Check sheet for the modelled part. Datum: model origin and axes. Units: mm. Give positions to 0.01 mm unless a question says otherwise; leave off trailing zeros. Order: outer loops, then holes, each group sorted by start corner. A loop starts at its lowest first (then second) coordinate and runs counter-clockwise, first axis right, second up. Notation, with made-up numbers: M 55,65.25 L 75,65.25 A18 ccw 75,98.25 Z; hole C 49.25,81 d10. An arc over 180 degrees is marked long. Answer in a Markdown table with one row per item. Add a question column.
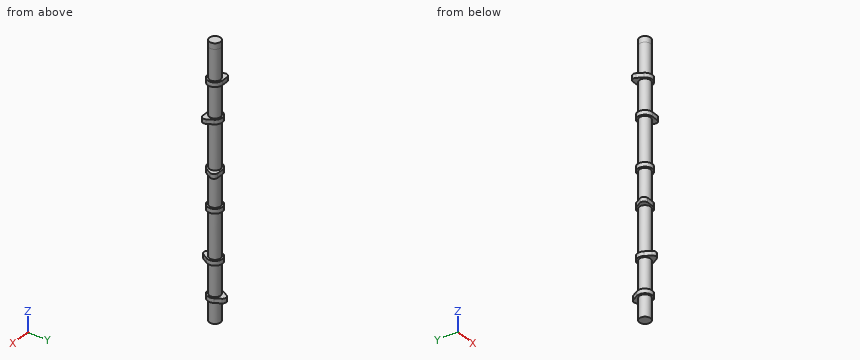
from build123d import *

# Parameters (mm, degrees)
BOSS_EXTRUDE1_DEPTH   = 3.81
BODY_MOVE_COPY2_ANGLE = 180
SKETCH2_R             = 9.5
BOSS_EXTRUDE2_DEPTH   = 146.05
LPATTERN1_COUNT       = 3
LPATTERN1_PITCH       = 146.05
BODY_MOVE_COPY3_ANGLE = 120
BODY_MOVE_COPY4_ANGLE = 120
BOSS_EXTRUDE3_START   = 27.94
SKETCH3_R             = 9.5
BOSS_EXTRUDE3_DEPTH   = 27.94
SKETCH4_R             = 9.5
CUT_EXTRUDE1_DEPTH    = 16.94
SKETCH5_R             = 9.5
BOSS_EXTRUDE4_DEPTH   = 10


with BuildPart() as part:
    # Sketch1 → Boss-Extrude1 (new, symmetric)
    with BuildSketch(Plane.XY):
        with BuildLine():
            Line((-5.499261314, 15.875), (-10.998522628, 6.35))
            ThreePointArc((-10.998522628, 6.35), (0, -12.7), (10.998522628, 6.35))
            Line((10.998522628, 6.35), (5.499261314, 15.875))
            ThreePointArc((5.499261314, 15.875), (0, 19.05), (-5.499261314, 15.875))
        make_face()
    extrude(amount=BOSS_EXTRUDE1_DEPTH, both=True)


with BuildPart() as body_2:
    # Body-Move_Copy1: copy of part
    add(part.part.moved(Location((0, 0, 60.96))))


with BuildPart() as body_2_1:
    # Body-Move_Copy2: moved
    add(body_2.part.rotate(Axis((0, 0, 0), (0, 0, 1)), BODY_MOVE_COPY2_ANGLE))


with BuildPart() as part_1:
    add(part.part)

    add(body_2_1.part)  # Boss-Extrude2 merges body 2
    # Sketch2 → Boss-Extrude2 (add)
    with BuildSketch(Plane(origin=(0, 0, -29.21), x_dir=(-1, 0, 0), z_dir=(0, 0, -1))):
        with Locations(Location((0, 0, 0), (0, 0, 180))):
            Circle(SKETCH2_R)
    extrude(amount=-BOSS_EXTRUDE2_DEPTH)


with BuildPart() as lpattern1_1:
    # LPattern1: pattern copy
    add(part_1.part.moved(Location(Vector(0, 0, 1) * (1 * LPATTERN1_PITCH))))


with BuildPart() as lpattern1_2:
    # LPattern1: pattern copy
    add(part_1.part.moved(Location(Vector(0, 0, 1) * (2 * LPATTERN1_PITCH))))


with BuildPart() as lpattern1_1_1:
    # Body-Move_Copy3: moved
    add(lpattern1_1.part.rotate(Axis((0, 0, 0), (0, 0, 1)), BODY_MOVE_COPY3_ANGLE))


with BuildPart() as lpattern1_2_1:
    # Body-Move_Copy4: moved
    add(lpattern1_2.part.rotate(Axis((0, 0, 0), (0, 0, -1)), BODY_MOVE_COPY4_ANGLE))


with BuildPart() as part_2:
    add(part_1.part)

    # Sketch3 → Boss-Extrude3 (add)
    with BuildSketch(Plane(origin=(0, 0, -29.21), x_dir=(-1, 0, 0), z_dir=(0, 0, -1)).offset(BOSS_EXTRUDE3_START)):
        with Locations(Location((0, 0, 0), (0, 0, 180))):
            Circle(SKETCH3_R)
    extrude(amount=-BOSS_EXTRUDE3_DEPTH)


with BuildPart() as lpattern1_2_2:
    add(lpattern1_2_1.part)

    # Combine1: union LPattern1_1, part
    add(lpattern1_1_1.part)
    add(part_2.part)

    # Sketch4 → Cut-Extrude1 (cut)
    with BuildSketch(Plane(origin=(0, 0, -57.15), x_dir=(-1, 0, 0), z_dir=(0, 0, -1))):
        Circle(SKETCH4_R)
    extrude(amount=-CUT_EXTRUDE1_DEPTH, mode=Mode.SUBTRACT)

    # Sketch5 → Boss-Extrude4 (add)
    with BuildSketch(Plane.XY.offset(408.94)):
        with Locations(Location((0, 0, 0), (0, 0, 180))):
            Circle(SKETCH5_R)
    extrude(amount=BOSS_EXTRUDE4_DEPTH)


solid = lpattern1_2_2.part
Q1. Thickness scan on probe 1 along Z at (x, y) = (3.5, 10); probe 2 along Z at (x, y) = (-11, -6.5); probe 3 along X at (y, z) = (0, 239). Record the ranges inside material, lowest first.
Q2. Go/stop test with flat-tipped pins: pin 1 (5 mm diameter, centred on y = 11, z = 95.5, fed in from +X); pin 2 (5 mm diameter, centred on x = -7.5, y = -13, fed in from -Z); pin 3 (6 mm diameter, centred on x = -6.5, z = 147, fed in from -Y). Record where each tip stops, or that it passes through.
Q3. Cross-section at A-A (z = 322). Record the boundary of the cut face in (x, y).
Values follow:
| question | item | result |
|---|---|---|
| 1 | probe 1 | -3.81 to 3.81, 57.15 to 64.77, 142.24 to 149.86, 203.2 to 210.82, 288.29 to 295.91, 349.25 to 356.87 |
| 1 | probe 2 | 142.24 to 149.86 |
| 1 | probe 3 | -9.5 to 9.5 |
| 2 | pin 1 | x = 4.24 |
| 2 | pin 2 | z = -3.81 |
| 2 | pin 3 | y = -12.7 |
| 3 | outline | C 0,0 d19 |
